Part model, mm, in its own coordinate system. A direction names the side the tool comes from. Round coordinates to 2 decimals unless told otherwise and drop trailing zeros. Write each loop counter-clockwise with the first axis right and the second up, starting at its lowest first coordinate (ties: lowest second). Pieces come first, ordered by that corner, then holes. Notation, with made-up numbers: M 73,84 L 79,84 A33 cw 79,116 Z; hole C 72,1 d10. An arc over 180 degrees is marked long. Answer as a JSON object with one key per item and string values. Group by question number.
1. Band-saw the part on B-B, the plane z = -29. Write the cut outline in (x, y) (3 decimals).
2. Drill centre lines: line 1 (Z direction, x = -163.75, y = 4.5) (3 decimals); line 2 (X direction, y = 9.5, z = -28). Where is each one in solid material? Low to high. Write a range as from..to.
3. Two-plate mould, pull along Z, no slides. Class faces 4 (the face through (-167, 15.875, -1)), 5 (the face through (-168, 0, -88.9)), 6 (the face through (-165.1, 0, -30)), 7 (the face through (-164, 0, 79.375)): +Z half, -Z half, draft (parallel to the pull), parting line (faces both ways), or undercut.
4. Band-saw the part on A-A, the plane y = 1.5. Write the cut outline in (x, z) (3 decimals).
5. Which spindle directions (+Z, -Z, +X, -X, +Y, -Y) get a long thin tool onto all of the face, cutting with end or side? Do faces 1 (the face through (-165.1, 0, 84)), 2 (the face through (-164, 0, -34.925)), 3 (the face through (-165.1, 0, -84)). Say none if no direction does.
6. Drop flat-ended pins along their axis: pin 1 (1.6 mm diameter, centred on x = -163.5, y = 2.5, fed in from +Z) (3 decimals); pin 2 (10.5 mm diameter, centred on y = -6, z = -31, fed in from +X) (3 decimals); pin 3 (3.5 mm diameter, centred on x = -163, y = -5, fed in from -Z) (3 decimals); pin 4 (1.5 mm diameter, centred on y = 2.5, z = -32, fed in from +X). Give the stop position or say it passes through.
from build123d import *

# Parameters (mm, degrees)
BOSS_EXTRUDE1_DEPTH      = 15.875
BOSS_EXTRUDE1_DEPTH_BACK = 15.875


with BuildPart() as part:
    # Sketch2 → Boss-Extrude1 (new, two sides: drawn at the far end of the back side and taken through both)
    with BuildSketch(Plane(origin=(0, 0, 0), x_dir=(1, 0, 0), z_dir=(0, 1, 0)).offset(-BOSS_EXTRUDE1_DEPTH_BACK)):
        Polygon((-171.45, 88.9), (-171.45, -88.9), (-165.1, -88.9), (-165.1, -79.375), (-161.925, -79.375), (-161.925, 25.4), (-165.1, 25.4), (-165.1, 34.925), (-161.925, 34.925), (-161.925, 79.375), (-165.1, 79.375), (-165.1, 88.9), align=None)
    extrude(amount=BOSS_EXTRUDE1_DEPTH + BOSS_EXTRUDE1_DEPTH_BACK)


solid = part.part
Worked answers:
{
 "1": {"outline": "M -171.45,-15.875 L -165.1,-15.875 L -165.1,15.875 L -171.45,15.875 Z"},
 "2": {"line 1": "z = -79.375..-34.925, -25.4..79.375", "line 2": "x = -171.45..-165.1"},
 "3": {"face 4": "draft", "face 5": "-Z half", "face 6": "undercut", "face 7": "+Z half"},
 "4": {"outline": "M -171.45,-88.9 L -165.1,-88.9 L -165.1,-79.375 L -161.925,-79.375 L -161.925,-34.925 L -165.1,-34.925 L -165.1,-25.4 L -161.925,-25.4 L -161.925,79.375 L -165.1,79.375 L -165.1,88.9 L -171.45,88.9 Z"},
 "5": {"face 1": "+Z, +X, +Y, -Y", "face 2": "+X, +Y, -Y", "face 3": "-Z, +X, +Y, -Y"},
 "6": {"pin 1": "stops at z = 79.375", "pin 2": "stops at x = -161.925", "pin 3": "stops at z = -79.375", "pin 4": "stops at x = -165.1"}
}
